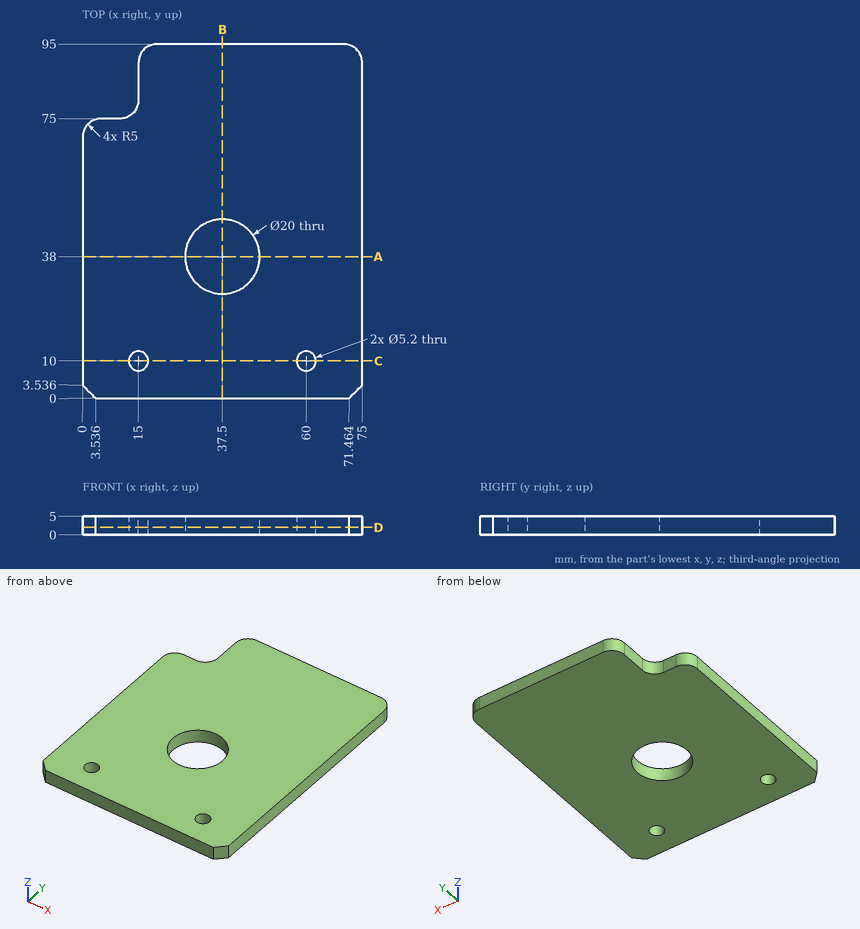
Geometry check sheet. Reference: drawing and pictorial views, mm from the part's lowest x, y, z. Give positions to 0.01 mm unless a question says otherwise; leave off trailing zeros. Order: outer loops, then holes, each group sorted by start corner. A loop starts at its lowest first (then second) coordinate and runs counter-clockwise, first axis right, second up.
1. Section check D-D, the plane z = 2.05. Enter the section's corners in (x, y) (1 decimal).
2. Section check C-C, the plane y = 10. Enter the section's corners in (x, z).
3. Section check A-A, the plane y = 38. Enter the section's corners in (x, z).
4. Gauge pin test, flat ends, axial feed: pin 1 Ø8.5 at (x, y) = (15, 10) entering from -Z; pin 2 Ø2.5 at (y, z) = (83.5, 2) entering from -X; pin 3 Ø1.5 at (x, z) = (7, 3) entering from +Y. Record the tip position at first contact, or that the pin passes through.
5. Thickness scan on L1, parallel to Y at x = 37.5, z = 3.3; L2, parallel to X at y = 8, z = 1.2; L3, parallel to X at y = 80, z = 3.2. Record the ranges inside material, lowest first.
6. Section check B-B, the plane x = 37.5. Enter the section's corners in (y, z), and give its area (3 significant figures).
Values follow:
1. outline: (0, 3.5) - (3.5, 0) - (71.5, 0) - (75, 3.5) - (75, 90) arc R5 ccw to (70, 95) - (20, 95) arc R5 ccw to (15, 90) - (15, 80) arc R5 cw to (10, 75) - (5, 75) arc R5 ccw to (0, 70) - close; hole circle Ø5.2 at (15, 10); hole circle Ø20 at (37.5, 38); hole circle Ø5.2 at (60, 10)
2. outline: (0, 0) - (12.4, 0) - (12.4, 5) - (0, 5) - close; (17.6, 0) - (57.4, 0) - (57.4, 5) - (17.6, 5) - close; (62.6, 0) - (75, 0) - (75, 5) - (62.6, 5) - close
3. outline: (0, 0) - (27.5, 0) - (27.5, 5) - (0, 5) - close; (47.5, 0) - (75, 0) - (75, 5) - (47.5, 5) - close
4. pin 1: stops at z = 0
4. pin 2: stops at x = 15
4. pin 3: stops at y = 75
5. L1: y = 0 to 28, 48 to 95
5. L2: x = 0 to 13.34, 16.66 to 58.34, 61.66 to 75
5. L3: x = 15 to 75
6. outline: (0, 0) - (28, 0) - (28, 5) - (0, 5) - close; (48, 0) - (95, 0) - (95, 5) - (48, 5) - close
6. area: 375 mm2
